For this review, take the finished solid that the model builds, in its own axes (mm). A direction names the side the tool comes from. Give positions to 0.01 mm unless a question says otherwise; leave off trailing zeros. Loops run counter-clockwise (first coordinate to the right, second up) from the corner with the lowest first, then second, coordinate; pieces in that order, holes last. Notation, with made-up numbers: (39, -22.5) - (94, -22.5) arc R23 cw to (94, -7.5) - close; hole circle Ø4 at (24.5, 2.25). An arc over 180 degrees is marked (long way). Use CSV: the item, a comma, the result in double quotes. Start each with the question number.
1. Take a section at C-C on x = 49. Give the boundary of the cut face in (y, z).
2. Mouldability with a two-part tool opening along Z and no side actions: class faces 5 (the flat face through (0, 4, 4.665)), 6 (the flat face through (17, 0, 20)), 7 (the cylindrical face through (-1.18, 4.44, 14.57)) as pulls with the +Z half, pulls with the -Z half, needs draft (parallel to the pull), parting line crosses it, or undercut.
3. For faces 1 (the flat face through (10, -4, 17)), 2 (the flat face through (23.786, -2, 17)), 3 (the flat face through (32, -2, 14.665)), 4 (the flat face through (21, 14, 17.665)), list the 3-axis set-ups (+Z, -Z, +X, -X, +Y, -Y) from which the entire face can be reached by the end or side of a thin tool; tool diameter is ignored.
4. Wall thickness on line 1 (X direction, y = 15.75, z = 14.5); line 2 (Z direction, x = 24.5, y = 13.5); line 3 (X direction, y = 12, z = 22): over which ranges is each line inside the solid? List them lowest first.
5. Take a section at A-A on y = -2.25. Give the boundary of the cut face in (x, z), plus the area to 3 significant figures.
6. Take a section at B-B on z = 7.75. Give the boundary of the cut face in (x, y).
7. Take a section at D-D on z = 21.75. Give the boundary of the cut face in (x, y).
8. For pin 1 (2 mm diameter, centred on x = 30.5, z = 22, fed in from -Y); pin 2 (2.5 mm diameter, centred on x = 3, y = -3, fed in from +Z); pin 3 (2.5 mm diameter, centred on x = 36.5, y = 2.5, fed in from +Z), all flat-tipped, find the tip position at first contact; note any pin that passes through.
```python
from build123d import *

# Parameters (mm, degrees)
SKETCH1_W             = 12
SKETCH1_H             = 12
SKETCH1_R             = 4
BOSS_EXTRUDE1_DEPTH   = 9
BOSS_EXTRUDE1_2_DEPTH = 9
BOSS_EXTRUDE1_3_DEPTH = 9
BOSS_EXTRUDE1_4_DEPTH = 9
BOSS_EXTRUDE1_5_DEPTH = 9
BOSS_EXTRUDE1_6_DEPTH = 9
SKETCH1_4_R           = 1.7
BOSS_EXTRUDE2_DEPTH   = 20
SKETCH2_W             = 2.2
SKETCH2_H             = 5.00000001
BOSS_EXTRUDE3_DEPTH   = 4
BOSS_EXTRUDE4_DEPTH   = 1
CUT_EXTRUDE1_DEPTH    = 1


with BuildPart() as part:
    # Sketch1 → Boss-Extrude1 (new body)
    with BuildSketch(Plane(origin=(0, 0, 0), x_dir=(1, 0, 0), z_dir=(0, 1, 0))):
        with Locations((6.88638754, -23.664883012)):
            Rectangle(SKETCH1_W, SKETCH1_H)
        with Locations((6.88638754, -23.664883012)):
            Circle(SKETCH1_R, mode=Mode.SUBTRACT)
    extrude(amount=BOSS_EXTRUDE1_DEPTH)



with BuildPart() as body_2:
    # Sketch1 → Boss-Extrude1 2 (new body)
    with BuildSketch(Plane(origin=(0, 0, 0), x_dir=(1, 0, 0), z_dir=(0, 1, 0))):
        with Locations((-0.31361246, -10.664883002)):
            Rectangle(SKETCH1_W, SKETCH1_H)
        with Locations((-0.31361246, -10.664883002)):
            Circle(SKETCH1_R, mode=Mode.SUBTRACT)
    extrude(amount=BOSS_EXTRUDE1_2_DEPTH)


with BuildPart() as body_3:
    # Sketch1 → Boss-Extrude1 3 (new body)
    with BuildSketch(Plane(origin=(0, 0, 0), x_dir=(1, 0, 0), z_dir=(0, 1, 0))):
        with Locations((14.08638754, -10.664883022)):
            Rectangle(SKETCH1_W, SKETCH1_H)
        with Locations((14.08638754, -10.664883022)):
            Circle(SKETCH1_R, mode=Mode.SUBTRACT)
    extrude(amount=BOSS_EXTRUDE1_3_DEPTH)


with BuildPart() as body_4:
    # Sketch1 → Boss-Extrude1 4 (new body)
    with BuildSketch(Plane(origin=(0, 0, 0), x_dir=(1, 0, 0), z_dir=(0, 1, 0))):
        with Locations((28.48638754, -10.664883043)):
            Rectangle(SKETCH1_W, SKETCH1_H)
        with Locations((28.48638754, -10.664883043)):
            Circle(SKETCH1_R, mode=Mode.SUBTRACT)
    extrude(amount=BOSS_EXTRUDE1_4_DEPTH)


with BuildPart() as body_5:
    # Sketch1 → Boss-Extrude1 5 (new body)
    with BuildSketch(Plane(origin=(0, 0, 0), x_dir=(1, 0, 0), z_dir=(0, 1, 0))):
        with Locations((21.28638754, -23.664883033)):
            Rectangle(SKETCH1_W, SKETCH1_H)
        with Locations((21.28638754, -23.664883033)):
            Circle(SKETCH1_R, mode=Mode.SUBTRACT)
    extrude(amount=BOSS_EXTRUDE1_5_DEPTH)


with BuildPart() as body_6:
    # Sketch1 → Boss-Extrude1 6 (new body)
    with BuildSketch(Plane(origin=(0, 0, 0), x_dir=(1, 0, 0), z_dir=(0, 1, 0))):
        with Locations((35.68638754, -23.664883053)):
            Rectangle(SKETCH1_W, SKETCH1_H)
        with Locations((35.68638754, -23.664883053)):
            Circle(SKETCH1_R, mode=Mode.SUBTRACT)
    extrude(amount=BOSS_EXTRUDE1_6_DEPTH)


with BuildPart() as part_1:
    add(part.part)

    add(body_2.part)  # Boss-Extrude2 merges body 2

    add(body_3.part)  # Boss-Extrude2 merges body 3

    add(body_4.part)  # Boss-Extrude2 merges body 4

    add(body_5.part)  # Boss-Extrude2 merges body 5

    add(body_6.part)  # Boss-Extrude2 merges body 6
    # Sketch1_4 → Boss-Extrude2 (add)
    with BuildSketch(Plane(origin=(0, 0, 0), x_dir=(1, 0, 0), z_dir=(0, 1, 0))):
        Polygon((0.38638754, -30.164883012), (0.38638754, -17.164883012), (-6.81361246, -17.164883002), (-6.81361246, -4.164883002), (-18.31361246, -4.164883002), (-18.31361246, -30.164883012), align=None)
        with Locations((-13.31361246, -17.164883007)):
            Circle(SKETCH1_4_R, mode=Mode.SUBTRACT)
        Polygon((29.18638754, -17.164883043), (27.78638754, -17.164883043), (27.78638754, -30.164883033), (29.18638754, -30.164883053), align=None)
        Polygon((20.58638754, -4.164883022), (20.58638754, -17.164883022), (21.98638754, -17.164883033), (21.98638754, -4.164883043), align=None)
        Polygon((14.78638754, -17.164883022), (13.38638754, -17.164883022), (13.38638754, -30.164883012), (14.78638754, -30.164883033), align=None)
        Polygon((7.58638754, -4.164883022), (6.18638754, -4.164883002), (6.18638754, -17.164883002), (7.58638754, -17.164883012), align=None)
        Polygon((6.18638754, -17.164883002), (6.18638754, -4.164883002), (2.18638754, -4.164883002), (2.18638754, -4.664883002), (5.68638754, -4.664883002), (5.68638754, -16.664883002), (-6.31361246, -16.664883002), (-6.31361246, -4.664883002), (-2.81361246, -4.664883002), (-2.81361246, -4.164883002), (-6.81361246, -4.164883002), (-6.81361246, -17.164883002), (0.38638754, -17.164883002), align=None)
        Polygon((7.58638754, -17.164883012), (6.18638754, -17.164883012), (0.38638754, -17.164883012), (0.38638754, -30.164883012), (4.38638754, -30.164883012), (4.38638754, -29.664883012), (0.88638754, -29.664883012), (0.88638754, -17.664883012), (12.88638754, -17.664883012), (12.88638754, -29.664883012), (9.38638754, -29.664883012), (9.38638754, -30.164883012), (13.38638754, -30.164883012), (13.38638754, -17.164883012), align=None)
        Polygon((11.58638754, -4.164883022), (7.58638754, -4.164883022), (7.58638754, -17.164883022), (13.38638754, -17.164883012), (14.78638754, -17.164883022), (20.58638754, -17.164883033), (20.58638754, -4.164883022), (16.58638754, -4.164883022), (16.58638754, -4.664883022), (20.08638754, -4.664883022), (20.08638754, -16.664883022), (8.08638754, -16.664883022), (8.08638754, -4.664883022), (11.58638754, -4.664883022), align=None)
        Polygon((34.98638754, -17.164883053), (29.18638754, -17.164883053), (29.18638754, -30.164883053), (33.18638754, -30.164883053), (33.18638754, -29.664883053), (29.68638754, -29.664883053), (29.68638754, -17.664883053), (41.68638754, -17.664883053), (41.68638754, -29.664883053), (38.18638754, -29.664883053), (38.18638754, -30.164883053), (42.18638754, -30.164883053), (42.18638754, -17.164883053), align=None)
        Polygon((21.98638754, -4.164883043), (21.98638754, -17.164883043), (27.78638754, -17.164883043), (29.18638754, -17.164883043), (34.98638754, -17.164883053), (34.98638754, -4.164883043), (30.98638754, -4.164883043), (30.98638754, -4.664883043), (34.48638754, -4.664883043), (34.48638754, -16.664883043), (22.48638754, -16.664883043), (22.48638754, -4.664883043), (25.98638754, -4.664883043), (25.98638754, -4.164883043), align=None)
        Polygon((20.58638754, -17.164883033), (14.78638754, -17.164883033), (14.78638754, -30.164883033), (18.78638754, -30.164883033), (18.78638754, -29.664883033), (15.28638754, -29.664883033), (15.28638754, -17.664883033), (27.28638754, -17.664883033), (27.28638754, -29.664883033), (23.78638754, -29.664883033), (23.78638754, -30.164883033), (27.78638754, -30.164883033), (27.78638754, -17.164883033), (21.98638754, -17.164883043), align=None)
        Polygon((34.98638754, -4.164883043), (34.98638754, -17.164883043), (42.18638754, -17.164883053), (42.18638754, -30.164883053), (53.68638754, -30.164883012), (53.68638754, -4.164883002), align=None)
        with Locations((48.68638754, -17.164883007)):
            Circle(SKETCH1_4_R, mode=Mode.SUBTRACT)
    extrude(amount=BOSS_EXTRUDE2_DEPTH)

    # Sketch2 → Boss-Extrude3 (add)
    with BuildSketch(Plane.XZ):
        with Locations((3.28638754, 17.164883007)):
            Rectangle(SKETCH2_W, SKETCH2_H)
        with Locations((10.48638754, 17.164883023)):
            Rectangle(SKETCH2_W, SKETCH2_H)
        with Locations((17.68638754, 17.164883038)):
            Rectangle(SKETCH2_W, SKETCH2_H)
        with Locations((24.88638754, 17.164883045)):
            Rectangle(SKETCH2_W, SKETCH2_H)
        with Locations((32.08638754, 17.164883007)):
            Rectangle(SKETCH2_W, SKETCH2_H)
    extrude(amount=BOSS_EXTRUDE3_DEPTH)

    # Sketch3 → Boss-Extrude4 (add)
    with BuildSketch(Plane.XZ):
        Polygon((-10.262781623, 27.059918831), (-8.715986751, 27.059918831), (-8.715986751, 26.734277806), (-9.977845725, 26.734277806), (-9.977845725, 25.757354729), (-8.715986751, 25.757354729), (-8.715986751, 25.431713703), (-9.977845725, 25.431713703), (-9.977845725, 23.884918831), (-10.262781623, 23.884918831), align=None)
        Polygon((-7.75623615, 27.059918831), (-7.169191879, 27.059918831), (-7.169191879, 23.884918831), (-7.454127777, 23.884918831), (-7.454127777, 26.734277806), (-7.942589315, 26.734277806), align=None)
    extrude(amount=-BOSS_EXTRUDE4_DEPTH)

    # Sketch3_2 → Cut-Extrude1 (cut)
    with BuildSketch(Plane.XZ):
        Polygon((-10.262781623, 27.059918831), (-8.715986751, 27.059918831), (-8.715986751, 26.734277806), (-9.977845725, 26.734277806), (-9.977845725, 25.757354729), (-8.715986751, 25.757354729), (-8.715986751, 25.431713703), (-9.977845725, 25.431713703), (-9.977845725, 23.884918831), (-10.262781623, 23.884918831), align=None)
        Polygon((-7.75623615, 27.059918831), (-7.169191879, 27.059918831), (-7.169191879, 23.884918831), (-7.454127777, 23.884918831), (-7.454127777, 26.734277806), (-7.942589315, 26.734277806), align=None)
    extrude(amount=-CUT_EXTRUDE1_DEPTH, mode=Mode.SUBTRACT)


solid = part_1.part
```
Check result:
1,outline,"(0, 4.16) - (20, 4.16) - (20, 15.49) - (0, 15.49) - close; (0, 18.84) - (20, 18.84) - (20, 30.16) - (0, 30.16) - close"
2,face 5,"pulls with the -Z half"
2,face 6,"needs draft"
2,face 7,"undercut"
3,face 1,"+Z, -Z, +X, -X, -Y"
3,face 2,"+Z, -Z, -Y"
3,face 3,"-Z, +X, -X, -Y"
3,face 4,"+Y"
4,line 1,"x = -18.31 to -6.31, 5.69 to 8.09, 20.09 to 22.49, 34.49 to 53.69"
4,line 2,"z = 4.16 to 4.66, 16.66 to 17.66, 29.66 to 30.16"
4,line 3,"x = -18.31 to 0.89, 12.89 to 15.29, 27.29 to 29.69, 41.69 to 53.69"
5,outline,"(2.19, 14.66) - (4.39, 14.66) - (4.39, 19.66) - (2.19, 19.66) - close; (9.39, 14.66) - (11.59, 14.66) - (11.59, 19.66) - (9.39, 19.66) - close; (16.59, 14.66) - (18.79, 14.66) - (18.79, 19.66) - (16.59, 19.66) - close; (23.79, 14.66) - (25.99, 14.66) - (25.99, 19.66) - (23.79, 19.66) - close; (30.99, 14.66) - (33.19, 14.66) - (33.19, 19.66) - (30.99, 19.66) - close"
5,area,"55.0 mm²"
6,outline,"(-18.31, 0) - (-3.05, 0) - (-3.05, 9) - (-6.31, 9) - (-6.31, 20) - (-18.31, 20) - close; (2.43, 0) - (11.35, 0) - (11.35, 9) - (8.09, 9) - (8.09, 20) - (5.69, 20) - (5.69, 9) - (2.43, 9) - close; (16.83, 0) - (25.75, 0) - (25.75, 9) - (22.49, 9) - (22.49, 20) - (20.09, 20) - (20.09, 9) - (16.83, 9) - close; (31.23, 0) - (53.69, 0) - (53.69, 20) - (34.49, 20) - (34.49, 9) - (31.23, 9) - close"
7,outline,"(-18.31, 0) - (3.37, 0) - (3.37, 9) - (0.89, 9) - (0.89, 20) - (-18.31, 20) - close; (10.4, 0) - (17.77, 0) - (17.77, 9) - (15.29, 9) - (15.29, 20) - (12.89, 20) - (12.89, 9) - (10.4, 9) - close; (24.8, 0) - (32.17, 0) - (32.17, 9) - (29.69, 9) - (29.69, 20) - (27.29, 20) - (27.29, 9) - (24.8, 9) - close; (39.2, 0) - (53.69, 0) - (53.69, 20) - (41.69, 20) - (41.69, 9) - (39.2, 9) - close"
8,pin 1,"stops at y = 0"
8,pin 2,"stops at z = 19.66"
8,pin 3,"stops at z = 29.66"
